Design review of the part built by this model. Coordinates are the model's own, in mm. A direction names the side the tool comes from. Give positions to 0.01 mm unless a question says otherwise; leave off trailing zeros. Write each loop counter-clockwise with the first axis right and the second up, starting at its lowest first coordinate (ties: lowest second). Pieces come first, ordered by that corner, then holes. Notation, with made-up numbers: M 39.5,6 L 89.5,6 A29 cw 89.5,42 Z; hole C 47,46.5 d1. An arc over 180 degrees is marked long. Answer in a Markdown table with one row per item.
```python
from build123d import *

# Parameters (mm, degrees)
SKETCH1_W        = 43
SKETCH1_H        = 21
BOARD_DEPTH      = 1.6
INDUCTOR_START   = 1.6
SKETCH2_W        = 12
SKETCH2_H        = 12
INDUCTOR_DEPTH   = 12.4
INPUT_CAP_START  = 1.6
SKETCH3_W        = 6
SKETCH3_H        = 7
INPUT_CAP_DEPTH  = 8
OUTPUT_CAP_START = 1.6
SKETCH4_W        = 6
SKETCH4_H        = 7
OUTPUT_CAP_DEPTH = 8


with BuildPart() as part:
    # Sketch1 → Board (new body)
    with BuildSketch(Plane(origin=(0, 0, 0), x_dir=(1, 0, 0), z_dir=(0, 1, 0))):
        Rectangle(SKETCH1_W, SKETCH1_H)
    extrude(amount=BOARD_DEPTH)

    # Sketch2 → Inductor (add)
    with BuildSketch(Plane(origin=(0, 0, 0), x_dir=(1, 0, 0), z_dir=(0, 1, 0)).offset(INDUCTOR_START)):
        Rectangle(SKETCH2_W, SKETCH2_H)
    extrude(amount=INDUCTOR_DEPTH)

    # Sketch3 → Input_Cap (add)
    with BuildSketch(Plane(origin=(0, 0, 0), x_dir=(1, 0, 0), z_dir=(0, 1, 0)).offset(INPUT_CAP_START)):
        with Locations((-16.5, 0)):
            Rectangle(SKETCH3_W, SKETCH3_H)
    extrude(amount=INPUT_CAP_DEPTH)

    # Sketch4 → Output_Cap (add)
    with BuildSketch(Plane(origin=(0, 0, 0), x_dir=(1, 0, 0), z_dir=(0, 1, 0)).offset(OUTPUT_CAP_START)):
        with Locations((15.5, 0)):
            Rectangle(SKETCH4_W, SKETCH4_H)
    extrude(amount=OUTPUT_CAP_DEPTH)


solid = part.part
```
1) To check wall thickness, follow probe 1 along X at (y, z) = (4.5, 2); probe 2 along Y at (x, z) = (-11, 5.75); probe 3 along Z at (x, y) = (17, 2). State the ranges of each line that lie inside material, in increasing order. Write a range as [from, to].
Geometry says:
| item | result |
|---|---|
| probe 1 | [-19.5, -13.5], [-6, 6], [12.5, 18.5] |
| probe 2 | [0, 1.6] |
| probe 3 | [-3.5, 3.5] |
2) Insertion check: P1, Ø7.5, axis at y = 6, z = 1, coming from the -X side; P2, Ø6.5, axis at x = 17, z = 1, coming from the +Y side; P3, Ø6, axis at x = -17, y = 7.5, coming from the +Z side. Each pin has a flat end and moves straight along its axis. Give the tip position at first contact, or say it passes through.
Geometry says:
| item | result |
|---|---|
| P1 | x = -19.5 |
| P2 | y = 9.6 |
| P3 | z = 3.5 |
3) The part is to be moulded in two halves that separate along X. For faces 6 (the face through (12.5, 6, 0)), 7 (the face through (-13.5, 6, 0)), 8 (the face through (-17, 6, 3.5)), 9 (the face through (18.5, 6, 0)), say which applies: released by +X, released by -X, zero draft, split by the parting line, or undercut.
Geometry says:
| item | result |
|---|---|
| face 6 | undercut |
| face 7 | undercut |
| face 8 | zero draft |
| face 9 | released by +X |
4) Add section B-B (x = -16). Write out the cut boundary in (y, z).
Geometry says:
| item | result |
|---|---|
| outline | M 0,-10.5 L 1.6,-10.5 L 1.6,-3.5 L 9.6,-3.5 L 9.6,3.5 L 1.6,3.5 L 1.6,10.5 L 0,10.5 Z |
5) Add section D-D (y = 11.75). Write out the cut boundary in (x, z).
Geometry says:
| item | result |
|---|---|
| outline | M -6,-6 L 6,-6 L 6,6 L -6,6 Z |
6) Add section A-A (y = 7.5). Write out the cut boundary in (x, z), and give its area (3 significant figures).
Geometry says:
| item | result |
|---|---|
| outline | M -19.5,-3.5 L -13.5,-3.5 L -13.5,3.5 L -19.5,3.5 Z; M -6,-6 L 6,-6 L 6,6 L -6,6 Z; M 12.5,-3.5 L 18.5,-3.5 L 18.5,3.5 L 12.5,3.5 Z |
| area | 228 mm^2 |
7) Add section C-C (z = 5). Write out the cut boundary in (x, y).
Geometry says:
| item | result |
|---|---|
| outline | M -21.5,0 L 21.5,0 L 21.5,1.6 L 6,1.6 L 6,14 L -6,14 L -6,1.6 L -21.5,1.6 Z |
8) For faces 1 (the face through (6, 8, 0)), 2 (the face through (-17, 6, -3.5)), 3 (the face through (0, 8, -6)), 4 (the face through (15, 6, -3.5)), 5 (the face through (15, 9.6, 0)), list the 3-axis set-ups (+Z, -Z, +X, -X, +Y, -Y) from which the entire face can be reached by the end or side of a thin tool; tool diameter is ignored.
Geometry says:
| item | result |
|---|---|
| face 1 | +Z, -Z, +Y |
| face 2 | -Z, -X, +Y |
| face 3 | -Z, +X, -X, +Y |
| face 4 | -Z, +X, +Y |
| face 5 | +Z, -Z, +X, +Y |
